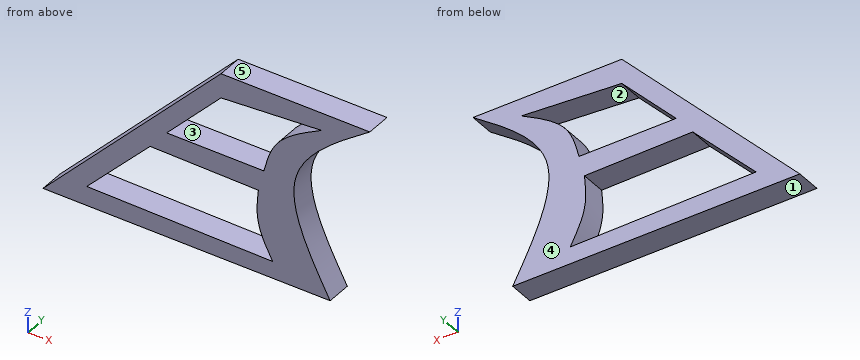
from build123d import *

# Parameters (mm, degrees)
F4_DEPTH = 4.4038286433
F1_DEPTH = 25.4
F3_DEPTH = 25.4


with BuildPart() as f4:
    # F0 (on Front) → F4 (new body)
    with BuildSketch(Plane.XZ):
        with BuildLine():
            Line((31.1220660806, 32.5515791774), (0, 0))
            Line((0, 0), (50.1943454146, 0))
            add(Edge.make_bspline(
                [(57.1354404092, 32.5515791774), (51.2567108227, 28.4945148136), (39.283604536, 20.231564454), (46.5140247255, 6.824346213), (50.1943454146, 0)],
                knots=[0, 0, 0, 0, 0.4909946095, 1, 1, 1, 1], degree=3))
            Line((57.1354404092, 32.5515791774), (31.1220660806, 32.5515791774))
        make_face()
    extrude(amount=F4_DEPTH)

    # F5 (on face) → F1 (cut)
    with BuildSketch(Plane.XZ.offset(4.4038286433)):
        with BuildLine():
            Line((48.6895032227, 29.4836014509), (31.1220660806, 28.2830670476))
            Line((31.1220660806, 28.2830670476), (21.6255090178, 18.3503097448))
            Line((21.6255090178, 18.3503097448), (38.6046469212, 18.3503097448))
            add(Edge.make_bspline(
                [(38.6046469212, 18.3503097448), (39.1462333934, 20.4801539657), (40.329776692, 25.1345605855), (45.7497139994, 27.9542141002), (48.6895032227, 29.4836014509)],
                knots=[0, 0, 0, 0, 0.4575973734, 1, 1, 1, 1], degree=3))
        make_face()
    extrude(amount=-F1_DEPTH, mode=Mode.SUBTRACT)

    # F2 (on face) → F3 (cut)
    with BuildSketch(Plane.XZ.offset(4.4038286433)):
        with BuildLine():
            Line((37.6483798027, 14.5543171093), (18.7260732055, 14.8174436763))
            Line((18.7260732055, 14.8174436763), (7.6506421901, 3.3673320431))
            Line((7.6506421901, 3.3673320431), (40.1368737221, 2.9665562324))
            add(Edge.make_bspline(
                [(40.1368737221, 2.9665562324), (39.0989015719, 4.8818670377), (37.0677097284, 8.6299096625), (37.4576869265, 12.6087358362), (37.6483798027, 14.5543171093)],
                knots=[0, 0, 0, 0, 0.5110162974, 1, 1, 1, 1], degree=3))
        make_face()
    extrude(amount=-F3_DEPTH, mode=Mode.SUBTRACT)


solid = f4.part
Model file for the job. Use its own axes, mm. Face numbers are marked on the shaded views. A direction names the side the tool comes from. Coordinates: 2 decimals unless noted, no trailing zeros. Order: outer loops, then holes, each group sorted by start corner. A loop starts at its lowest first (then second) coordinate and runs counter-clockwise, first axis right, second up. Notation, with made-up numbers: (24.25, -7.5) -> (71.25, -7.5) arc R22 ccw to (71.25, 4.5) -> close; hole circle Ø11 at (52, -17). An arc over 180 degrees is marked (long way). Return JSON: item names as keys, results as strings. Group by question number.
Item 1: Tool access for the marked faces 1 and 2: list every direction of +Z, -Z, +X, -X, +Y, -Y with a clear straight run to the whole face (end or side of a thin tool).
Item 2: Pull direction Z, two halves, no side cores. Call the marked faces 3, 4 and 5: pulls with the +Z half, pulls with the -Z half, needs draft (parallel to the pull), parting line crosses it, or undercut.
Item 3: Saw through at C-C on y = -3.4. State how many separate pieces and enclosed holes the cut face has, then the cut area to 3 significant figures.
Item 4: Saw through at D-D on x = 7. Write the cut outline in (y, z), then the cut area to 3 significant figures.
Item 5: Saw through at A-A on x = 18. Write the cut outline in (y, z), then the cut area to 3 significant figures.
Item 6: Saw through at B-B on x = 30. Write the cut outline in (y, z), then the cut area to 3 significant figures.
Item 7: Flat gauge pin, fed straight in: P1, Ø1.5, axis at x = 23.5, z = 24.5, coming from the +Y side. Where does the tip first touch, or does it go through?
Item 8: Wall check: line 1 along Z through (x, y) = (24, -1.5); line 2 along Z through (x, y) = (40, -2.05); line 3 along Z through (x, y) = (20, -0.95). Give the ranges that are in metal, low to high. Write a range as [from, to].
Values found:
{
 "1": {"face 1": "-Z, +X, -X, +Y, -Y", "face 2": "+Y, -Y"},
 "2": {"face 3": "undercut", "face 4": "needs draft", "face 5": "pulls with the +Z half"},
 "3": {"separate pieces": "1", "enclosed holes": "2", "area": "590 mm2"},
 "4": {"outline": "(-4.4, 0) -> (0, 0) -> (0, 7.32) -> (-4.4, 7.32) -> close", "area": "32.2 mm2"},
 "5": {"outline": "(-4.4, 0) -> (0, 0) -> (0, 3.24) -> (-4.4, 3.24) -> close; (-4.4, 14.07) -> (0, 14.07) -> (0, 18.83) -> (-4.4, 18.83) -> close", "area": "35.2 mm2"},
 "6": {"outline": "(-4.4, 0) -> (0, 0) -> (0, 3.09) -> (-4.4, 3.09) -> close; (-4.4, 14.66) -> (0, 14.66) -> (0, 18.35) -> (-4.4, 18.35) -> close; (-4.4, 27.11) -> (0, 27.11) -> (0, 31.38) -> (-4.4, 31.38) -> close", "area": "48.7 mm2"},
 "7": {"P1": "stops at y = 0"},
 "8": {"line 1": "z = [0, 3.17], [14.74, 18.35], [20.83, 25.1]", "line 2": "z = [0, 2.97], [3.22, 22.6], [28.89, 32.55]", "line 3": "z = [0, 3.21], [14.8, 20.92]"}
}
